Source: three-view drawing plus pictorial views. Frame: mm from the lowest corner of the part. A direction names the side the tool comes from. Round coordinates to 2 decimals unless told otherwise and drop trailing zeros. Write each loop counter-clockwise with the first axis right and the second up, starting at its lowest first coordinate (ties: lowest second). Pieces come first, ordered by that corner, then holes. Notation, with made-up numbers: M 6.5,53 L 13.5,53 A18 ccw 13.5,67 Z; hole C 36.5,57.5 d11. An arc over 180 degrees is marked long. Answer as CSV lines item,"result". Start each with the question number.
Q1. Section query B-B on z = 112.5. Output: boundary loops of the cut face in (x, y), and give its area (3 significant figures).
Q2. Section query C-C on x = 15. Output: boundary loops of the cut face in (y, z), and give its area (3 significant figures).
Q3. Section query A-A on x = 35. Output: boundary loops of the cut face in (y, z).
Q4. Section query D-D on y = 28. Output: boundary loops of the cut face in (x, z).
Q5. Reachability of the marked faces 1, 2, 3 and 4 from +Z, -Z, +X, -X, +Y, -Y: full face, straight path, thin tool, end or side. Return the list, or none.
Q6. First-contact query: pin 1 (5 mm diameter, centred on x = 5, z = 58, fed in from +Y); pin 2 (4 mm diameter, centred on x = 30.5, y = 66, fed in from +Z); pin 3 (1.5 mm diameter, centred on x = 6, z = 100, fed in from -Y). Flat tips, straight axial feed; report the tip coordinate or a pass-through.
Q7. Ray query, probe 1 along Y at (x, z) = (15, 2); probe 2 along Z at (x, y) = (35, 46.5); probe 3 along Z at (x, y) = (15, 64). Return the intervals inside material, ascending.
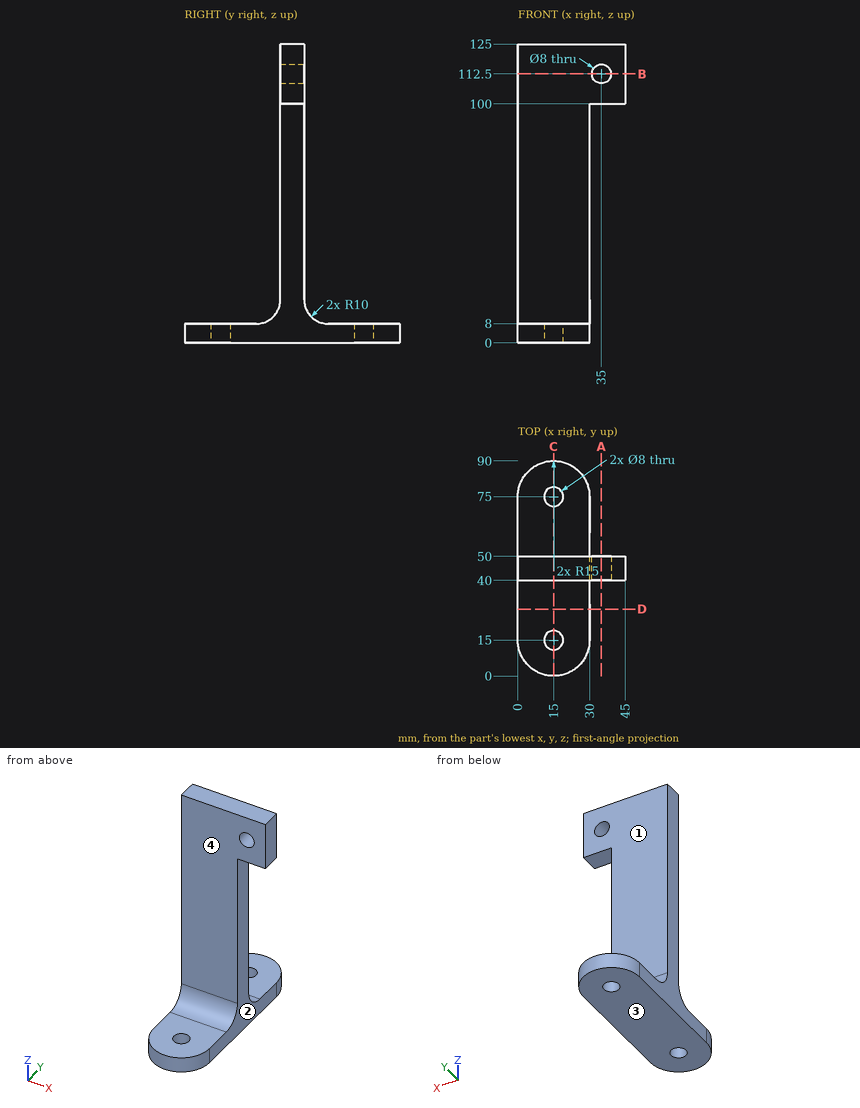
Entries:
1,outline,"M 0,40 L 31,40 L 31,50 L 0,50 Z; M 39,40 L 45,40 L 45,50 L 39,50 Z"
1,area,"370 mm^2"
2,outline,"M 0,0 L 11,0 L 11,8 L 0,8 Z; M 19,0 L 71,0 L 71,8 L 60,8 A10 cw 50,18 L 50,125 L 40,125 L 40,18 A10 cw 30,8 L 19,8 Z; M 79,0 L 90,0 L 90,8 L 79,8 Z"
2,area,"1,800 mm^2"
3,outline,"M 40,100 L 50,100 L 50,108.5 L 40,108.5 Z; M 40,116.5 L 50,116.5 L 50,125 L 40,125 Z"
4,outline,"M 0,0 L 30,0 L 30,8 L 0,8 Z"
5,face 1,"+Z, +X, -X, +Y"
5,face 2,"-Z, +X, +Y, -Y"
5,face 3,"-Z, +X, -X, +Y, -Y"
5,face 4,"+Z, +X, -X, -Y"
6,pin 1,"stops at y = 50"
6,pin 2,"stops at z = 8"
6,pin 3,"stops at y = 40"
7,probe 1,"y = 0 to 11, 19 to 71, 79 to 90"
7,probe 2,"z = 100 to 108.5, 116.5 to 125"
7,probe 3,"z = 0 to 8"
